```python
from build123d import *

# Parameters (mm, degrees)
SKETCH1_W           = 6.35
SKETCH1_H           = 19.05
SKETCH2_W           = 4.7625
SKETCH2_H           = 3.175
SKETCH2_W_2         = 0.762
SKETCH2_H_2         = 0.762
BOSS_EXTRUDE1_DEPTH = 101.6
SKETCH6_W           = 0.762
SKETCH6_H           = 0.762
CUT_EXTRUDE2_DEPTH  = 6.35
LPATTERN1_COUNT     = 2
LPATTERN1_PITCH     = 3.175
LPATTERN1_COL_COUNT = 2
LPATTERN1_COL_PITCH = 3.175


with BuildPart() as part:
    # Sketch1 → Revolve1 (revolve)
    with BuildSketch(Plane.XY):
        with Locations((-3.175, 9.525)):
            Rectangle(SKETCH1_W, SKETCH1_H)
    revolve(axis=Axis((0, 19.05, 0), (0, -1, 0)))

    # Sketch2 → Boss-Extrude1 (add)
    with BuildSketch(Plane(origin=(0, 19.05, 0), x_dir=(1, 0, 0), z_dir=(0, 1, 0))):
        with Locations((-1.49225, 0)):
            Rectangle(SKETCH2_W, SKETCH2_H)
        Rectangle(SKETCH2_W_2, SKETCH2_H_2, mode=Mode.SUBTRACT)
    boss_extrude1 = extrude(amount=BOSS_EXTRUDE1_DEPTH)

    # Sketch6 → Cut-Extrude2 (cut)
    with BuildSketch(Plane(origin=(0, 19.05, 0), x_dir=(1, 0, 0), z_dir=(0, 1, 0))):
        Rectangle(SKETCH6_W, SKETCH6_H)
    cut_extrude2 = extrude(amount=-CUT_EXTRUDE2_DEPTH, mode=Mode.SUBTRACT)

    # LPattern1: Boss-Extrude1, Cut-Extrude2 ×2
    with Locations(*[(0, 0, -i * LPATTERN1_PITCH) for i in range(1, LPATTERN1_COUNT)]):
        add(boss_extrude1)
        add(cut_extrude2, mode=Mode.SUBTRACT)

    # LPattern1 col: Boss-Extrude1, Cut-Extrude2 ×2
    with Locations(*[(0, 0, i * LPATTERN1_COL_PITCH) for i in range(1, LPATTERN1_COL_COUNT)]):
        add(boss_extrude1)
        add(cut_extrude2, mode=Mode.SUBTRACT)

    # Sketch4 → 1_8 NPT Tapped Hole1 (revolve, cut)
    with BuildSketch(Plane(origin=(0, 0, 0), x_dir=(0, 0, -1), z_dir=(1, 0, 0))):
        Polygon((0, 0), (0, 18.408468714), (4.2164, 15.875), (4.2164, 6.858), (4.537401096, 6.858), (4.7427388, 0), align=None)
    revolve(axis=Axis((0, -6.35, 0), (0, 1, 0)), mode=Mode.SUBTRACT)


solid = part.part
```
Here's how the part is built. I have some questions about the finished solid (model axes, mm). A direction names the side the tool comes from. Round coordinates to 2 decimals unless told otherwise and drop trailing zeros. Write each loop counter-clockwise with the first axis right and the second up, starting at its lowest first coordinate (ties: lowest second). Pieces come first, ordered by that corner, then holes.
Q1. If we mould it in two halves opening along Z, with no side actions, what happens to faces 6 (the cylindrical face through (-4.18, 11.3, 0.55)), 7 (the flat face through (-2, 69, 4.762)), 8 (the flat face through (0.889, 69, 0))? For each: +Z half, -Z half, draft (parallel to the pull), parting line (faces both ways), or undercut.
Q2. Which directions (+Z, -Z, +X, -X, +Y, -Y) give clear straight access to the entire face, cutting with the end or side of a thin tool? Please do faces 1 (the flat face through (-2, 120.65, 0)), 2 (the conical face through (-1.39, 3.38, -4.43)), 3 (the flat face through (-2, 69, -4.762)), 4 (the cylindrical face through (1.38, 9.66, 6.2)), 5 (the flat face through (-3.874, 69, 0)).
Q3. If we section it at A-A on y = 59.5: Write out the boundary of the cut face in (x, z).
Q4. Will these pins go through, and if not, where does the flat tip stop? P1, Ø1, axis at x = -1, y = 58, coming from the -Z side; P2, Ø5, axis at y = 51.5, z = -3, coming from the +X side; P3, Ø4, axis at x = -2, y = 51, coming from the +Z side.
Q5. Please list where these lines run through material, in increasing order: probe 1 along Z at (x, y) = (0, 12); probe 2 along Y at (x, z) = (4.5, -4).
Answer below:
1. face 6: undercut
1. face 7: +Z half
1. face 8: draft
2. face 1: +Z, -Z, +X, -X, +Y
2. face 2: -Y
2. face 3: -Z, +X, -X, +Y
2. face 4: +Y, -Y
2. face 5: +Z, -Z, -X, +Y
3. outline: (-3.87, -4.76) - (0.89, -4.76) - (0.89, 4.76) - (-3.87, 4.76) - close; hole (-0.38, -3.56) - (0.38, -3.56) - (0.38, -2.79) - (-0.38, -2.79) - close; hole (-0.38, -0.38) - (0.38, -0.38) - (0.38, 0.38) - (-0.38, 0.38) - close; hole (-0.38, 2.79) - (0.38, 2.79) - (0.38, 3.56) - (-0.38, 3.56) - close
4. P1: stops at z = -4.76
4. P2: stops at x = 0.89
4. P3: stops at z = 4.76
5. probe 1: z = -6.35 to -4.22, 4.22 to 6.35
5. probe 2: y = 0 to 19.05
